from build123d import *

# Parameters (mm, degrees)
SKETCH1_R           = 5.07
BOSS_EXTRUDE1_DEPTH = 76.9
SKETCH2_R           = 1.97
CUT_EXTRUDE1_DEPTH  = 15.2
CHAMFER2_SIZE       = 0.3
CUT_EXTRUDE2_START  = -15.2
SKETCH3_R           = 1.97
CUT_EXTRUDE2_DEPTH  = 15.2
CHAMFER3_SIZE       = 0.3


with BuildPart() as part:
    # Sketch1 → Boss-Extrude1 (new body)
    with BuildSketch(Plane(origin=(0, 0, 0), x_dir=(1, 0, 0), z_dir=(0, 1, 0))):
        with Locations(Location((0, 0, 0), (0, 0, 270))):
            Circle(SKETCH1_R)
    extrude(amount=BOSS_EXTRUDE1_DEPTH)

    # Sketch2 → Cut-Extrude1 (cut)
    with BuildSketch(Plane(origin=(0, 76.9, 0), x_dir=(1, 0, 0), z_dir=(0, 1, 0))):
        with Locations(Location((0, 0, 0), (0, 0, 270))):
            Circle(SKETCH2_R)
    extrude(amount=-CUT_EXTRUDE1_DEPTH, mode=Mode.SUBTRACT)

    # Chamfer2
    chamfer2_edges = [part.edges().sort_by_distance(p)[0] for p in [
        (0, 76.9, -1.97),
    ]]
    chamfer(chamfer2_edges, length=CHAMFER2_SIZE)

    # Sketch3 → Cut-Extrude2 (cut)
    with BuildSketch(Plane(origin=(0, 0, 0), x_dir=(-1, 0, 0), z_dir=(0, -1, 0)).offset(CUT_EXTRUDE2_START)):
        with Locations(Location((0, 0, 0), (0, 0, 270))):
            Circle(SKETCH3_R)
    extrude(amount=CUT_EXTRUDE2_DEPTH, mode=Mode.SUBTRACT)

    # Chamfer3
    chamfer3_edges = [part.edges().sort_by_distance(p)[0] for p in [
        (0, 0, -1.97),
    ]]
    chamfer(chamfer3_edges, length=CHAMFER3_SIZE)


solid = part.part
Verification items for the finished model (mm, model axes). A direction names the side the tool comes from. Give positions to 0.01 mm unless a question says otherwise; leave off trailing zeros. Write each loop counter-clockwise with the first axis right and the second up, starting at its lowest first coordinate (ties: lowest second). Pieces come first, ordered by that corner, then holes. Notation, with made-up numbers: M 9.5,76.25 L 57.5,76.25 A25 ccw 57.5,94.25 Z; hole C -31,-20 d4. An arc over 180 degrees is marked long. Write item = value, one per line.
(1) Access from +Z, -Z, +X, -X, +Y, -Y to the whole of each face (thin tool, end or side, straight path). Record for faces 1 (the face through (-1.1, 76.9, 2.2)), 2 (the face through (0, 15.2, 0)), 3 (the face through (-1.923, 69.254, -0.427)).
Found:
face_1 = +Z, -Z, +X, -X, +Y
face_2 = -Y
face_3 = +Y
(2) Draft check along Z on faces 4 (the face through (4.275, 37.912, 2.726)), 5 (the face through (0, 61.7, 0)), 6 (the face through (-1.1, 0, 2.2)). Enter one of: released by +Z, released by -Z, zero draft, split by the parting line, or undercut.
Found:
face_4 = split by the parting line
face_5 = undercut
face_6 = zero draft
(3) Sectioned sample at B-B (z = 0). Record the cut outline in (x, y).
Found:
outline = M -5.07,0 L -2.27,0 L -1.97,0.3 L -1.97,15.2 L 1.97,15.2 L 1.97,0.3 L 2.27,0 L 5.07,0 L 5.07,76.9 L 2.27,76.9 L 1.97,76.6 L 1.97,61.7 L -1.97,61.7 L -1.97,76.6 L -2.27,76.9 L -5.07,76.9 Z
(4) Sectioned sample at C-C (y = 9.5). Record the cut outline in (x, z), then the cut area to 3 significant figures.
Found:
outline = C 0,0 d10.14; hole C 0,0 d3.94
area = 68.6 mm2
(5) Material ranges on line 1 (X direction, y = 12, z = 0); line 2 (Y direction, x = 0, z = -1.25); line 3 (X direction, y = 6.5, z = -1.5), recorded low to high.
Found:
line_1 = -5.07 to -1.97, 1.97 to 5.07
line_2 = 15.2 to 61.7
line_3 = -4.84 to -1.28, 1.28 to 4.84
(6) Sectioned sample at D-D (y = 45). Record the cut outline in (x, z), then the cut area to 3 significant figures.
Found:
outline = C 0,0 d10.14
area = 80.8 mm2
(7) Sectioned sample at A-A (x = 0). Record the cut outline in (y, z), then the cut area to 3 significant figures.
Found:
outline = M 0,-5.07 L 76.9,-5.07 L 76.9,-2.27 L 76.6,-1.97 L 61.7,-1.97 L 61.7,1.97 L 76.6,1.97 L 76.9,2.27 L 76.9,5.07 L 0,5.07 L 0,2.27 L 0.3,1.97 L 15.2,1.97 L 15.2,-1.97 L 0.3,-1.97 L 0,-2.27 Z
area = 660 mm2
(8) Go/stop test with flat-tipped pins: pin 1 Ø1.2 at (x, z) = (0, 0.5) entering from -Y; pin 2 Ø4 at (y, z) = (37, 3) entering from -X; pin 3 Ø4 at (y, z) = (63.5, 2.5) entering from +X. Record where each tip stops, or that it passes through.
Found:
pin_1 = 15.2
pin_2 = -4.97
pin_3 = 5.05
